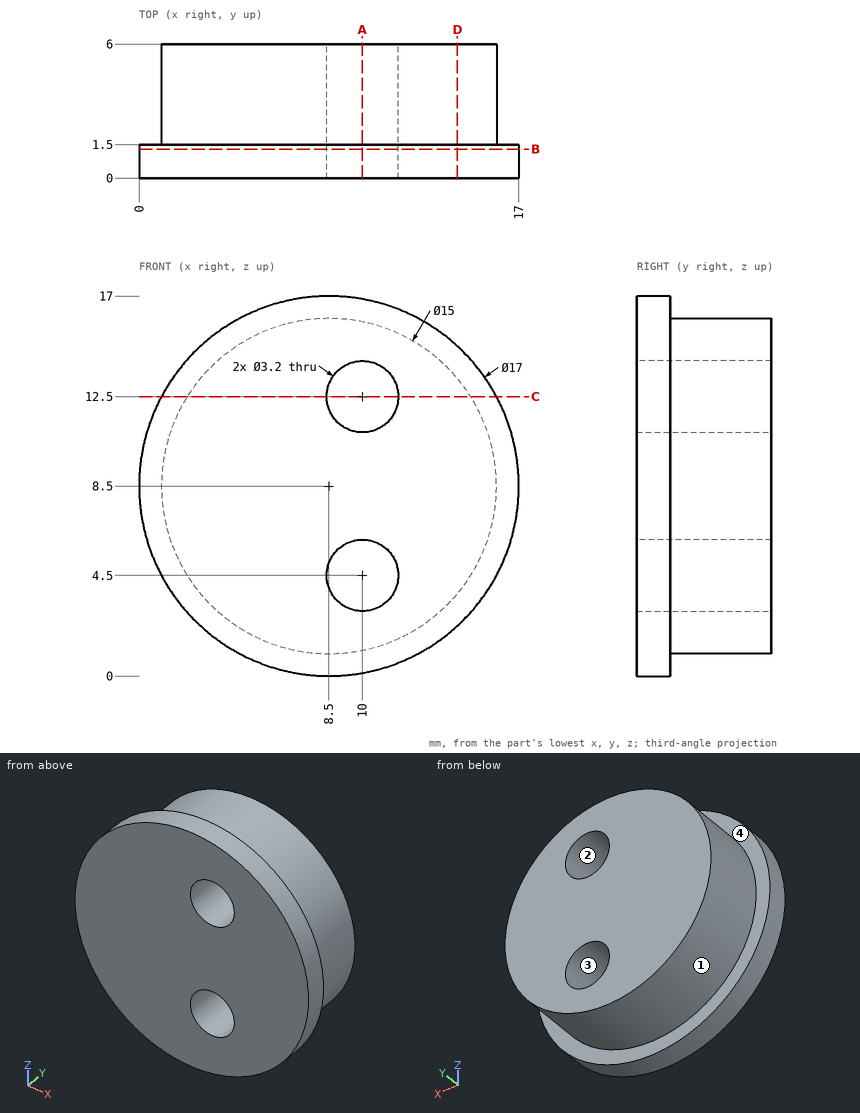
Design review of the part shown in the three views and the two pictorial views. Dimensions are in mm from the part's minimum x, y and z. Round coordinates to 2 decimals unless told otherwise and drop trailing zeros. Write each loop counter-clockwise with the first axis right and the second up, starting at its lowest first coordinate (ties: lowest second). Pieces come first, ordered by that corner, then holes. Notation, with made-up numbers: M 66.5,-19.5 L 118.5,-19.5 A22 cw 118.5,19.5 Z; hole C 2.25,40 d9. An arc over 180 degrees is marked long. One line per item, written item: value. Start each with the question number.
1. Clearance check with flat-ended pins moving along their axes: P1, Ø1.5, axis at x = 7.5, y = 4.5, coming from the -Z side; P2, Ø1, axis at x = 9.5, y = 2.5, coming from the +Z side; P3, Ø1.5, axis at y = 1, z = 6.5, coming from the +X side. State where each tip first meets the part, or that it passes through.
2. Take a section at B-B on y = 1.3. State the section outline as (x, z) points.
3. To check wall thickness, follow probe 1 along Z at (x, y) = (9.75, 3.3); probe 2 along X at (y, z) = (1.2, 5.25); probe 3 along X at (y, z) = (3.6, 11.25). State the ranges of each line that lie inside material, in increasing order. Write a range as from..to.
4. Take a section at C-C on z = 12.5. State the section outline as (x, y) points, then the cut area to 3 significant figures.
5. Take a section at D-D on x = 14.25. State the section outline as (y, z) points.
6. Draft analysis for pull direction X (two halves, no side actions). For the marked faces 1, 2, 3 and 4, state which applies: pulls with the +X half, pulls with the -X half, needs draft (parallel to the pull), parting line crosses it, or undercut.
7. Take a section at A-A on x = 10. State the section outline as (y, z) points.
Computed:
1. P1: stops at z = 1
1. P2: stops at z = 15.98
1. P3: stops at x = 16.91
2. outline: C 8.5,8.5 d17; hole C 10,4.5 d3.2; hole C 10,12.5 d3.2
3. probe 1: z = 1.1..2.92, 6.08..10.92, 14.08..15.9
3. probe 2: x = 0.65..8.59, 11.41..16.35
3. probe 3: x = 1.52..9, 11..15.48
4. outline: M 1,0 L 8.4,0 L 8.4,6 L 2.16,6 L 2.16,1.5 L 1,1.5 Z; M 11.6,0 L 16,0 L 16,1.5 L 14.84,1.5 L 14.84,6 L 11.6,6 Z
4. area: 60.4 mm²
5. outline: M 0,2.24 L 1.5,2.24 L 1.5,3.68 L 6,3.68 L 6,13.32 L 1.5,13.32 L 1.5,14.76 L 0,14.76 Z
6. face 1: parting line crosses it
6. face 2: undercut
6. face 3: undercut
6. face 4: needs draft
7. outline: M 0,0.13 L 1.5,0.13 L 1.5,1.15 L 6,1.15 L 6,2.9 L 0,2.9 Z; M 0,6.1 L 6,6.1 L 6,10.9 L 0,10.9 Z; M 0,14.1 L 6,14.1 L 6,15.85 L 1.5,15.85 L 1.5,16.87 L 0,16.87 Z
